Input: part model. Units: mm. Frame: model coordinates. A direction names the side the tool comes from. Give positions to 0.01 mm unless a question says otherwise; leave off trailing zeros. Write each loop counter-clockwise with the first axis right and the second up, starting at its lowest first coordinate (ties: lowest second). Pieces come first, ordered by that corner, then holes. Notation, with made-up numbers: (67, 63.25) -> (123, 63.25) arc R26 cw to (123, 87.25) -> close; hole circle Ø5 at (59.5, 32.25). An arc over 180 degrees is marked (long way). Return JSON: item names as keys, results as strings. Group by question number.
Item 1: Section C-C, the plane y = 156.5. Return loops of the section in (x, z) (3 decimals), then the cut area to 3 significant figures.
Item 2: Pin query (flat end, axial travel): P1, Ø5, axis at x = 38, y = 125.5, coming from the +Z side; P2, Ø1.5, axis at y = 156, z = -1, coming from the +X side; P3, Ø1.6, axis at x = 33, z = -1, coming from the +Y side; P4, Ø1, axis at y = 75.5, z = -1.5, coming from the +X side. Return the tip coordinate at first contact, or that it passes through.
Item 3: Set-up query: faces 5 (the face through (79.543, -15.163, -1.565)), 6 (the face through (-43.537, 117.415, -1.61)). Return all of +Z, -Z, +X, -X, +Y, -Y with unobstructed straight access to the full face (end or side cutting, diameter ignored); none if empty.
Item 4: Mould query, pull axis Y, two halves, no side actions, for faces 1 (the face through (-79.698, -15.007, -1.565)), 2 (the face through (57.737, 84.199, -1.61)), 3 (the face through (43.13, 118.18, -1.61)), 4 (the face through (0.385, 197.883, -1.61)). Classes: released by +Y, released by -Y, zero draft, split by the parting line, or undercut.
Item 5: Line query: line 1 (Y direction, x = 0, z = -1.5); line 2 (X direction, y = 35.5, z = -1.35); line 3 (X direction, y = 77.5, z = -1.3). Output: solid intervals per line, ascending. Write a range as [from, to].
Item 6: Section A-A, the plane y = 130. Return loops of the section in (x, z) (3 decimals), then the cut area to 3 significant figures.
Item 7: Section B-B, the plane z = -1.3. Count the separate pieces of the cut face and the enclosed holes in it, then the cut area to 3 significant figures.
from build123d import *

# Parameters (mm, degrees)
AM_1014_TI_PLATE_BOTTOM_4_AM_0001_ARTEME_START = -3.175
AM_1014_TI_PLATE_BOTTOM_4_AM_0001_AR_2_R       = 1.5875
AM_1014_TI_PLATE_BOTTOM_4_AM_0001_AR_2_R_2     = 1.906243542
AM_1014_TI_PLATE_BOTTOM_4_AM_0001_AR_2_R_3     = 3.175
AM_1014_TI_PLATE_BOTTOM_4_AM_0001_ARTEME_DEPTH = 3.175
BOSS_EXTRUDE1_DEPTH                            = 3.175
FILLET1_R                                      = 10
FILLET2_R                                      = 10


# Read off the part's stored shape, not the designer's step: AM_1014_TI_PLATE_BOTTOM<4>@AM_0001_ARTEMECH
with BuildPart() as part:
    # AM_1014_TI_PLATE_BOTTOM_4_AM_0001_AR 2 → AM_1014_TI_PLATE_BOTTOM<4>@AM_0001_ARTEMECH (new body)
    with BuildSketch(Plane.XY.offset(AM_1014_TI_PLATE_BOTTOM_4_AM_0001_ARTEME_START)):
        with BuildLine():
            Line((-82.55, 70.885609673), (-82.55, -18.014390327))
            Line((-82.55, -18.014390327), (82.55, -18.014390327))
            Line((82.55, -18.014390327), (82.55, 70.885609673))
            Line((82.55, 70.885609673), (22.446426721, 184.373331383))
            ThreePointArc((22.446426721, 184.373331383), (0, 197.885609673), (-22.446426721, 184.373331383))
            Line((-22.446426721, 184.373331383), (-82.55, 70.885609673))
        make_face()
        with Locations((-77.7875, -0.234390327)):
            Circle(AM_1014_TI_PLATE_BOTTOM_4_AM_0001_AR_2_R, mode=Mode.SUBTRACT)
        with Locations((-63.5, 1.035609673)):
            Circle(AM_1014_TI_PLATE_BOTTOM_4_AM_0001_AR_2_R_2, mode=Mode.SUBTRACT)
        with Locations((-77.7875, 17.545609673)):
            Circle(AM_1014_TI_PLATE_BOTTOM_4_AM_0001_AR_2_R, mode=Mode.SUBTRACT)
        with Locations((-77.7875, 35.325609673)):
            Circle(AM_1014_TI_PLATE_BOTTOM_4_AM_0001_AR_2_R, mode=Mode.SUBTRACT)
        with Locations((-11.416585625, 1.035609673)):
            Circle(AM_1014_TI_PLATE_BOTTOM_4_AM_0001_AR_2_R_2, mode=Mode.SUBTRACT)
        with Locations((-77.7875, 53.105609673)):
            Circle(AM_1014_TI_PLATE_BOTTOM_4_AM_0001_AR_2_R, mode=Mode.SUBTRACT)
        with Locations((-77.7875, 64.535609673)):
            Circle(AM_1014_TI_PLATE_BOTTOM_4_AM_0001_AR_2_R, mode=Mode.SUBTRACT)
        with BuildLine():
            Line((-25.4, 42.310609673), (-25.4, 51.835609673))
            ThreePointArc((-25.4, 51.835609673), (-27.25987194, 56.325737733), (-31.75, 58.185609673))
            Line((-31.75, 58.185609673), (-31.651036949, 58.185609673))
            ThreePointArc((-31.651036949, 58.185609673), (-27.160908889, 56.325737733), (-25.301036949, 51.835609673))
            Line((-25.301036949, 51.835609673), (-25.301036949, 42.310609673))
            ThreePointArc((-25.301036949, 42.310609673), (-24.37110098, 40.065545642), (-22.126036949, 39.135609673))
            Line((-22.126036949, 39.135609673), (-22.225, 39.135609673))
            ThreePointArc((-22.225, 39.135609673), (-24.470064031, 40.065545642), (-25.4, 42.310609673))
        make_face(mode=Mode.SUBTRACT)
        with Locations((-21.166666667, 47.762966307)):
            Circle(AM_1014_TI_PLATE_BOTTOM_4_AM_0001_AR_2_R, mode=Mode.SUBTRACT)
        with BuildLine():
            ThreePointArc((-11.2, 77.174125728), (-9.5, 78.874125728), (-7.8, 77.174125728))
            Line((-7.8, 77.174125728), (-7.8, 64.474125728))
            ThreePointArc((-7.8, 64.474125728), (-9.5, 62.774125728), (-11.2, 64.474125728))
            Line((-11.2, 64.474125728), (-11.2, 77.174125728))
        make_face(mode=Mode.SUBTRACT)
        with BuildLine():
            ThreePointArc((-1.7, 85.174125728), (0, 86.874125728), (1.7, 85.174125728))
            Line((1.7, 85.174125728), (1.7, 56.474125728))
            ThreePointArc((1.7, 56.474125728), (0, 54.774125728), (-1.7, 56.474125728))
            Line((-1.7, 56.474125728), (-1.7, 85.174125728))
        make_face(mode=Mode.SUBTRACT)
        with Locations((77.7875, -0.234390327)):
            Circle(AM_1014_TI_PLATE_BOTTOM_4_AM_0001_AR_2_R, mode=Mode.SUBTRACT)
        with Locations((77.7875, 17.545609673)):
            Circle(AM_1014_TI_PLATE_BOTTOM_4_AM_0001_AR_2_R, mode=Mode.SUBTRACT)
        with Locations((77.7875, 35.325609673)):
            Circle(AM_1014_TI_PLATE_BOTTOM_4_AM_0001_AR_2_R, mode=Mode.SUBTRACT)
        with Locations((21.166666667, 47.762966307)):
            Circle(AM_1014_TI_PLATE_BOTTOM_4_AM_0001_AR_2_R, mode=Mode.SUBTRACT)
        with BuildLine():
            ThreePointArc((7.8, 77.174125728), (9.5, 78.874125728), (11.2, 77.174125728))
            Line((11.2, 77.174125728), (11.2, 64.474125728))
            ThreePointArc((11.2, 64.474125728), (9.5, 62.774125728), (7.8, 64.474125728))
            Line((7.8, 64.474125728), (7.8, 77.174125728))
        make_face(mode=Mode.SUBTRACT)
        with Locations((77.7875, 53.105609673)):
            Circle(AM_1014_TI_PLATE_BOTTOM_4_AM_0001_AR_2_R, mode=Mode.SUBTRACT)
        with Locations((77.7875, 64.535609673)):
            Circle(AM_1014_TI_PLATE_BOTTOM_4_AM_0001_AR_2_R, mode=Mode.SUBTRACT)
        with BuildLine():
            ThreePointArc((-28.80539088, 145.230757697), (-24.546211379, 148.463135508), (-19.3281535, 147.296624336))
            ThreePointArc((-19.3281535, 147.296624336), (-17.639343437, 146.086441824), (-15.875, 144.989303103))
            ThreePointArc((-15.875, 144.989303103), (-13.550738686, 142.665041789), (-12.7, 139.490041789))
            Line((-12.7, 139.490041789), (-12.7, 87.395609673))
            ThreePointArc((-12.7, 87.395609673), (-14.559871939, 82.905481612), (-19.05, 81.045609673))
            Line((-19.05, 81.045609673), (-52.249574284, 81.045609673))
            ThreePointArc((-52.249574284, 81.045609673), (-57.689898641, 84.120648468), (-57.861180964, 90.3675401))
            Line((-57.861180964, 90.3675401), (-28.80539088, 145.230757697))
        make_face(mode=Mode.SUBTRACT)
        with Locations((0, 172.485609673)):
            Circle(AM_1014_TI_PLATE_BOTTOM_4_AM_0001_AR_2_R_3, mode=Mode.SUBTRACT)
        with BuildLine():
            ThreePointArc((12.7, 139.490041789), (13.550738686, 142.665041789), (15.875, 144.989303103))
            ThreePointArc((15.875, 144.989303103), (17.639343437, 146.086441824), (19.3281535, 147.296624336))
            ThreePointArc((19.3281535, 147.296624336), (24.546211379, 148.463135508), (28.80539088, 145.230757697))
            Line((28.80539088, 145.230757697), (57.861180964, 90.3675401))
            ThreePointArc((57.861180964, 90.3675401), (57.689898641, 84.120648468), (52.249574284, 81.045609673))
            Line((52.249574284, 81.045609673), (19.05, 81.045609673))
            ThreePointArc((19.05, 81.045609673), (14.559871939, 82.905481612), (12.7, 87.395609673))
            Line((12.7, 87.395609673), (12.7, 139.490041789))
        make_face(mode=Mode.SUBTRACT)
    extrude(amount=AM_1014_TI_PLATE_BOTTOM_4_AM_0001_ARTEME_DEPTH)

    # Sketch2 → Boss-Extrude1 (add)
    with BuildSketch(Plane.XY):
        Polygon((-34.947413532, 60.439294241), (-28.081020706, 36.459737757), (-19.207528438, 36.459737757), (-20.497701901, 40.965420465), (-23.644274572, 43.537404208), (-23.644274572, 54.206722292), (-24.602914342, 57.554587336), (-28.081020706, 60.39756411), align=None)
    extrude(amount=-BOSS_EXTRUDE1_DEPTH)

    # Fillet1
    fillet1_edges = [part.edges().sort_by_distance(p)[0] for p in [
        (-82.55, -18.014390327, -1.5875),
        (82.55, -18.014390327, -1.5875),
    ]]
    fillet(fillet1_edges, radius=FILLET1_R)

    # Fillet2
    fillet2_edges = [part.edges().sort_by_distance(p)[0] for p in [
        (82.55, 70.885609673, -1.5875),
        (-82.55, 70.885609673, -1.5875),
    ]]
    fillet(fillet2_edges, radius=FILLET2_R)


solid = part.part
Answer below:
{
 "1": {"outline": "(-37.208, -3.175) -> (37.208, -3.175) -> (37.208, 0) -> (-37.208, 0) -> close", "area": "236 mm2"},
 "2": {"P1": "stops at z = 0", "P2": "stops at x = 37.87", "P3": "stops at y = 165.96", "P4": "stops at x = 80.37"},
 "3": {"face 5": "+Z, -Z, +X, -Y", "face 6": "+Z, -Z"},
 "4": {"face 1": "released by -Y", "face 2": "undercut", "face 3": "undercut", "face 4": "released by +Y"},
 "5": {"line 1": "y = [-18.01, 54.77], [86.87, 169.31], [175.66, 197.89]", "line 2": "x = [-82.55, -79.37], [-76.21, 76.21], [79.37, 82.55]", "line 3": "x = [-79.05, -11.17], [-7.83, -1.7], [1.7, 7.83], [11.17, 79.05]"},
 "6": {"outline": "(-51.243, -3.175) -> (-36.872, -3.175) -> (-36.872, 0) -> (-51.243, 0) -> close; (-12.7, -3.175) -> (12.7, -3.175) -> (12.7, 0) -> (-12.7, 0) -> close; (36.872, -3.175) -> (51.243, -3.175) -> (51.243, 0) -> (36.872, 0) -> close", "area": "172 mm2"},
 "7": {"separate pieces": "1", "enclosed holes": "20", "area": "22,400 mm2"}
}
